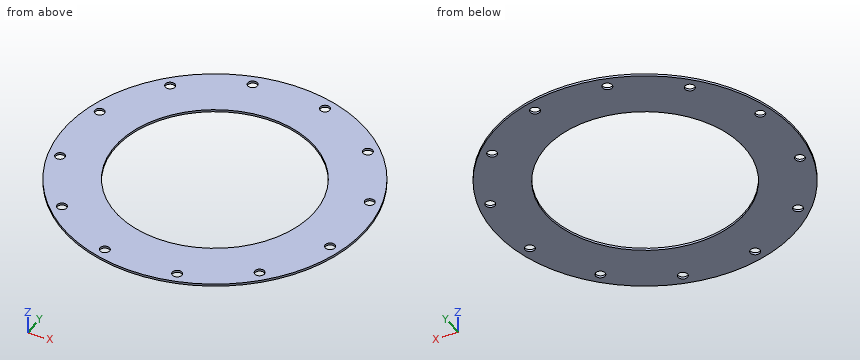
Autodesk Inventor part; units mm, degrees
ref_plane "YZ Plane" through (0, 0, 0) normal (1, 0, 0) x (0, 1, 0)
ref_plane "XZ Plane" through (0, 0, 0) normal (0, 1, 0) x (-1, 0, 0)
ref_plane "XY Plane" through (0, 0, 0) normal (0, 0, 1) x (1, 0, 0)
sketch "スケッチ4" plane through (0, 0, 1) normal (0, 0, 1) x (1, 0, 0)
  circle A0 centre (16.1762, 60.3704) radius 2.15
  circle A1 centre (-16.1762, 60.3704) radius 2.15
  circle A2 centre (0, 0) radius 67.5
  circle A3 centre (-16.1762, 60.3704) radius 5
  circle A4 centre (16.1762, 60.3704) radius 5
  circle A5 centre (0, 0) radius 62.5
  point P0 (-11.2987, 61.4702)
  point P1 (11.2987, 61.4702)
  point P2 (17.4703, 65.2)
  point P3 (-17.4703, 65.2)
sketch "スケッチ1" plane through (0, 0, 0) normal (0, 0, 1) x (1, 0, 0)
  circle A0 centre (0, 0) radius 67.5
  dimension "d0" = 135
extrude "プレート1" add sketch "スケッチ1" along normal blind 1
sketch "スケッチ2" plane through (0, 0, 1) normal (0, 0, 1) x (1, 0, 0)
  circle A0 centre (0, 0) radius 44.5
  dimension "d2" = 89
extrude "押し出し1" cut sketch "スケッチ2" against normal through all
sketch "スケッチ3" plane through (0, 0, 1) normal (0, 0, 1) x (1, 0, 0)
  circle A0 centre (0, 0) radius 62.5
  point P0 (16.1762, 60.3704)
  point P1 (-16.1762, 60.3704)
  point P2 (-44.1942, 44.1942)
  point P3 (-60.3704, 16.1762)
  point P4 (-60.3704, -16.1762)
  point P5 (-44.1942, -44.1942)
  point P6 (-16.1762, -60.3704)
  point P7 (16.1762, -60.3704)
  point P8 (44.1942, -44.1942)
  point P9 (60.3704, -16.1762)
  point P10 (60.3704, 16.1762)
  point P11 (44.1942, 44.1942)
  dimension "d5" = 125
  dimension "d8" = 360
  dimension "d23" = 0
hole "穴1" at (16.1762, 60.3704, 1) at (-16.1762, 60.3704, 1) at (-44.1942, 44.1942, 1) at (-60.3704, 16.1762, 1) at (-60.3704, -16.1762, 1) at (-44.1942, -44.1942, 1) at (-16.1762, -60.3704, 1) at (16.1762, -60.3704, 1) at (44.1942, -44.1942, 1) at (60.3704, -16.1762, 1) at (60.3704, 16.1762, 1) at (44.1942, 44.1942, 1) direction (0, 0, -1) diameter 4.3 end through all
equation "\"d15\" = Thickness"
equation "\"d1\" = Thickness"
equation "\"BendRadius\" = Thickness"
equation "\"BendReliefWidth\" = Thickness"
equation "\"BendReliefDepth\" = 0.5 * Thickness"
equation "\"CornerReliefSize\" = 4 * Thickness"
equation "\"MinimumRemnant\" = 2 * Thickness"
equation "\"TransitionRadius\" = BendRadius"
equation "\"JacobiRadiusSize\" = BendRadius"
equation "\"GapSize\" = Thickness"
properties part number "unit-plate3" material "CFRP"
Geometry check sheet. Reference: the model listing, model coordinates, mm. Give positions to 0.01 mm unless a question says otherwise; leave off trailing zeros. Loops run counter-clockwise (first coordinate to the right, second up) from the corner with the lowest first, then second, coordinate; pieces in that order, holes last.
(1) Section check D-D on y = 48. Record the cut outline in (x, z), then the cut area to 3 significant figures.
From the geometry:
outline: (-47.46, 0) - (47.46, 0) - (47.46, 1) - (-47.46, 1) - close
area: 94.9 mm2
(2) Thickness scan on L1, parallel to Y at x = -58.5, z = 0.15; L2, parallel to X at y = -15.5, z = 0.95; L3, parallel to Y at x = -27.5, z = 0.3. Record the ranges inside material, lowest first.
From the geometry:
L1: y = -33.67 to -17.24, -15.12 to 15.12, 17.24 to 33.67
L2: x = -65.7 to -62.41, -58.33 to -41.71, 41.71 to 58.33, 62.41 to 65.7
L3: y = -61.64 to -34.99, 34.99 to 61.64
(3) Section check C-C on z = 0.5. Count the separate pieces of the cut face and the enclosed holes in it, then the cut area to 3 significant figures.
From the geometry:
separate pieces: 1
enclosed holes: 13
area: 7,920 mm2
(4) Section check A-A on y = 0. Record the cut outline in (x, z), then the cut area to 3 significant figures.
From the geometry:
outline: (-67.5, 0) - (-44.5, 0) - (-44.5, 1) - (-67.5, 1) - close; (44.5, 0) - (67.5, 0) - (67.5, 1) - (44.5, 1) - close
area: 46.0 mm2
(5) Depth check by flat-ended pin: pin 1 Ø7 at (x, y) = (-60.37, -16.18) entering from +Z; pin 2 Ø12 at (x, y) = (15, -32) entering from +Z. Enter the tip coordinate at first touch or a pass-through.
From the geometry:
pin 1: stops at z = 1
pin 2: passes through
